from build123d import *
from build123d.topology import SkipClean

# Parameters (mm, degrees)
ESQUISSE1_W             = 7
ESQUISSE1_H             = 8
ESQUISSE1_W_2           = 5
BOSS_EXTRU_1_DEPTH      = 1.5
ESQUISSE2_R             = 1
BOSS_EXTRU_2_DEPTH      = 0.8
ESQUISSE3_W             = 1.5
ESQUISSE3_H             = 10.5
ENL_V_MAT_EXTRU_1_DEPTH = 28.5


with BuildPart() as part:
    # Esquisse1 → Boss.-Extru.1 (new body)
    # profile 1 of 5: a face of its own
    with BuildSketch(Plane.XY):
        Polygon((-54.543024121, 30.316995205), (-54.543024121, 22.316995205), (-53.543024121, 22.316995205), (-53.543024121, 31.316995205), (-82.043024121, 31.316995205), (-82.043024121, 22.316995205), (-80.043024121, 22.316995205), (-80.043024121, 30.316995205), (-75.043024121, 30.316995205), (-75.043024121, 22.316995205), (-61.543024121, 22.316995205), (-61.543024121, 30.316995205), align=None)
        with BuildLine():
            ThreePointArc((-69.793024121, 26.816995205), (-67.793024121, 28.816995205), (-65.793024121, 26.816995205))
            ThreePointArc((-65.793024121, 26.816995205), (-67.793024121, 24.816995205), (-69.793024121, 26.816995205))
        make_face(mode=Mode.SUBTRACT)
    # profile 2 of 5: a face of its own
    with BuildSketch(Plane.XY):
        Polygon((-55.643024121, 20.316995205), (-54.543024121, 20.316995205), (-54.543024121, 22.316995205), (-61.543024121, 22.316995205), (-61.543024121, 20.316995205), (-60.443024121, 20.316995205), (-60.443024121, 12.816995205), (-59.443024121, 11.816995205), (-56.643024121, 11.816995205), (-55.643024121, 12.816995205), align=None)
        with BuildLine():
            ThreePointArc((-59.043024121, 17.816995205), (-58.043024121, 18.816995205), (-57.043024121, 17.816995205))
            Line((-57.043024121, 17.816995205), (-57.043024121, 15.316995205))
            ThreePointArc((-57.043024121, 15.316995205), (-58.043024121, 14.316995205), (-59.043024121, 15.316995205))
            Line((-59.043024121, 15.316995205), (-59.043024121, 17.816995205))
        make_face(mode=Mode.SUBTRACT)
    # profile 3 of 5: a face of its own
    with BuildSketch(Plane.XY):
        Polygon((-75.043024121, 20.316995205), (-75.043024121, 22.316995205), (-80.043024121, 22.316995205), (-80.043024121, 20.316995205), (-78.943024121, 20.316995205), (-78.943024121, 12.616995205), (-78.143024121, 11.816995205), (-76.943024121, 11.816995205), (-76.143024121, 12.616995205), (-76.143024121, 20.316995205), align=None)
        with BuildLine():
            ThreePointArc((-78.143024121, 16.916995205), (-77.543024121, 17.516995205), (-76.943024121, 16.916995205))
            Line((-76.943024121, 16.916995205), (-76.943024121, 14.916995205))
            ThreePointArc((-76.943024121, 14.916995205), (-77.543024121, 14.316995205), (-78.143024121, 14.916995205))
            Line((-78.143024121, 14.916995205), (-78.143024121, 16.916995205))
        make_face(mode=Mode.SUBTRACT)
    # profile 4 of 5: a face of its own
    with BuildSketch(Plane.XY):
        with Locations((-58.043024121, 26.316995205)):
            Rectangle(ESQUISSE1_W, ESQUISSE1_H)
        with BuildLine():
            ThreePointArc((-58.943024121, 26.816995205), (-57.943024121, 27.816995205), (-56.943024121, 26.816995205))
            ThreePointArc((-56.943024121, 26.816995205), (-57.943024121, 25.816995205), (-58.943024121, 26.816995205))
        make_face(mode=Mode.SUBTRACT)
    # profile 5 of 5: a face of its own
    with BuildSketch(Plane.XY):
        with Locations((-77.543024121, 26.316995205)):
            Rectangle(ESQUISSE1_W_2, ESQUISSE1_H)
        with BuildLine():
            ThreePointArc((-76.643024121, 26.816995205), (-77.643024121, 25.816995205), (-78.643024121, 26.816995205))
            ThreePointArc((-78.643024121, 26.816995205), (-77.643024121, 27.816995205), (-76.643024121, 26.816995205))
        make_face(mode=Mode.SUBTRACT)
    extrude(amount=BOSS_EXTRU_1_DEPTH)

    # Esquisse2 → Boss.-Extru.2 (add)
    # profile 1 of 2: a face of its own
    with SkipClean():  # the faces are left unmerged after this step: merging them gives an invalid solid
        with BuildSketch(Plane.XY.offset(1.5)):
            Polygon((-80.043024121, 22.316995205), (-80.043024121, 20.316995205), (-78.943024121, 20.316995205), (-78.943024121, 12.616995205), (-78.143024121, 11.816995205), (-76.943024121, 11.816995205), (-76.143024121, 12.616995205), (-76.143024121, 20.316995205), (-75.043024121, 20.316995205), (-75.043024121, 22.316995205), (-75.043024121, 30.316995205), (-80.043024121, 30.316995205), align=None)
            with BuildLine():
                ThreePointArc((-78.143024121, 16.916995205), (-77.543024121, 17.516995205), (-76.943024121, 16.916995205))
                Line((-76.943024121, 16.916995205), (-76.943024121, 14.916995205))
                ThreePointArc((-76.943024121, 14.916995205), (-77.543024121, 14.316995205), (-78.143024121, 14.916995205))
                Line((-78.143024121, 14.916995205), (-78.143024121, 16.916995205))
            make_face(mode=Mode.SUBTRACT)
            with Locations((-77.643024121, 26.816995205)):
                Circle(ESQUISSE2_R, mode=Mode.SUBTRACT)
        # profile 2 of 2: a face of its own
        with BuildSketch(Plane.XY.offset(1.5)):
            Polygon((-61.543024121, 22.316995205), (-61.543024121, 20.316995205), (-60.443024121, 20.316995205), (-60.443024121, 12.816995205), (-59.443024121, 11.816995205), (-56.643024121, 11.816995205), (-55.643024121, 12.816995205), (-55.643024121, 20.316995205), (-54.543024121, 20.316995205), (-54.543024121, 22.316995205), (-54.543024121, 30.316995205), (-61.543024121, 30.316995205), align=None)
            with BuildLine():
                ThreePointArc((-59.043024121, 17.816995205), (-58.043024121, 18.816995205), (-57.043024121, 17.816995205))
                Line((-57.043024121, 17.816995205), (-57.043024121, 15.316995205))
                ThreePointArc((-57.043024121, 15.316995205), (-58.043024121, 14.316995205), (-59.043024121, 15.316995205))
                Line((-59.043024121, 15.316995205), (-59.043024121, 17.816995205))
            make_face(mode=Mode.SUBTRACT)
            with Locations((-57.943024121, 26.816995205)):
                Circle(ESQUISSE2_R, mode=Mode.SUBTRACT)
        extrude(amount=BOSS_EXTRU_2_DEPTH)

    # Esquisse3 → Enlèv. mat.-Extru.1 (cut)
    with SkipClean():  # the faces are left unmerged after this step: merging them gives an invalid solid
        with BuildSketch(Plane.ZY.offset(82.043024121)):
            with Locations((0.75, 17.066995205)):
                Rectangle(ESQUISSE3_W, ESQUISSE3_H)
        extrude(amount=-ENL_V_MAT_EXTRU_1_DEPTH, mode=Mode.SUBTRACT)
    add(part.part.scale(1), mode=Mode.REPLACE)  # the faces are merged on a copy


solid = part.part
Geometry check sheet. Reference: the model listing, model coordinates, mm. A direction names the side the tool comes from. Round coordinates to 2 decimals unless told otherwise and drop trailing zeros. Loops run counter-clockwise (first coordinate to the right, second up) from the corner with the lowest first, then second, coordinate; pieces in that order, holes last. Notation, with made-up numbers: (81.5, 6) - (128.5, 6) arc R27 cw to (128.5, 42) - close; hole circle Ø2 at (43.5, -35). An arc over 180 degrees is marked (long way). Answer as CSV lines item,"result".
(1) Release check for a two-part mould opening along X. For faces 4 (the face through (-56.15, 12.31, 1.89)), 5 (the face through (-58.065, 18.817, 1.894)), 6 (the face through (-78, 18, 1.5)) record: released by +X, released by -X, zero draft, split by the parting line, or undercut.
Output values:
face 4,"released by +X"
face 5,"undercut"
face 6,"zero draft"
(2) Cross-section at D-D, the plane y = 30. Enter the section's corners in (x, z).
Output values:
outline,"(-82.04, 0) - (-53.54, 0) - (-53.54, 1.5) - (-54.54, 1.5) - (-54.54, 2.3) - (-61.54, 2.3) - (-61.54, 1.5) - (-75.04, 1.5) - (-75.04, 2.3) - (-80.04, 2.3) - (-80.04, 1.5) - (-82.04, 1.5) - close"
(3) Cross-section at C-C, the plane x = -67.25. Enter the section's corners in (y, z).
Output values:
outline,"(22.32, 0) - (24.89, 0) - (24.89, 1.5) - (22.32, 1.5) - close; (28.74, 0) - (31.32, 0) - (31.32, 1.5) - (28.74, 1.5) - close"
(4) Material ranges on line 1 along X through (y, z) = (16.75, 1.7); line 2 along X through (y, z) = (17.25, 2.25); line 3 along X through (y, z) = (20.5, 2.25), recorded low to high.
Output values:
line 1,"x = -78.94 to -78.14, -76.94 to -76.14, -60.44 to -59.04, -57.04 to -55.64"
line 2,"x = -78.94 to -78.04, -77.04 to -76.14, -60.44 to -59.04, -57.04 to -55.64"
line 3,"x = -80.04 to -75.04, -61.54 to -54.54"
(5) Cross-section at A-A, the plane y = 21.5. Enter the section's corners in (x, z).
Output values:
outline,"(-80.04, 1.5) - (-75.04, 1.5) - (-75.04, 2.3) - (-80.04, 2.3) - close; (-61.54, 1.5) - (-54.54, 1.5) - (-54.54, 2.3) - (-61.54, 2.3) - close"
(6) Depth check by flat-ended pin: pin 1 Ø2.5 at (x, y) = (-57.94, 26.82) entering from +Z; pin 2 Ø0.6 at (y, z) = (17, 2) entering from +X; pin 3 Ø1.2 at (x, z) = (-62, 1) entering from -Y; pin 4 Ø2.5 at (x, y) = (-78.5, 16.5) entering from -Z. Enter the tip coordinate at first touch or a pass-through.
Output values:
pin 1,"stops at z = 2.3"
pin 2,"stops at x = -55.64"
pin 3,"stops at y = 22.32"
pin 4,"stops at z = 1.5"
(7) Set-up check for faces 1 (the face through (-68, 22.317, 1)), 2 (the face through (-59.95, 12.324, 1.894)), 3 (the face through (-58.021, 14.317, 1.894)): record each of +Z, -Z, +X, -X, +Y, -Y from which the full face is reachable in a straight line by a thin tool's end or side.
Output values:
face 1,"-Z, +X, -X, -Y"
face 2,"+Z, -Z, -Y"
face 3,"+Z, -Z"
(8) Cross-section at B-B, the plane z = 1.95. Give the number of separate pieces and of enclosed holes in the cut face, and give its area (3 significant figures).
Output values:
separate pieces,"2"
enclosed holes,"4"
area,"165 mm²"
